from build123d import *

# Parameters (mm, degrees)
SKETCH1_W           = 25.4
SKETCH1_H           = 50.8
SKETCH1_W_2         = 19.05
SKETCH1_H_2         = 44.45
BOSS_EXTRUDE1_DEPTH = 317.5
SKETCH2_R           = 1.905
CUT_EXTRUDE1_DEPTH  = 322.789030267
SKETCH3_R           = 2.1971
SKETCH3_R_2         = 2.8067
CUT_EXTRUDE2_DEPTH  = 322.789030267


with BuildPart() as part:
    # Sketch1 → Boss-Extrude1 (new, symmetric)
    with BuildSketch(Plane.XY):
        Rectangle(SKETCH1_W, SKETCH1_H)
        Rectangle(SKETCH1_W_2, SKETCH1_H_2, mode=Mode.SUBTRACT)
    extrude(amount=BOSS_EXTRUDE1_DEPTH, both=True)

    # Sketch2 → Cut-Extrude1 (cut, through all)
    with BuildSketch(Plane(origin=(0, 25.4, 0), x_dir=(1, 0, 0), z_dir=(0, 1, 0))):
        with Locations(Location((0, -120.1166, 0), (0, 0, 270))):
            Circle(SKETCH2_R)
        with Locations(Location((0, -94.7166, 0), (0, 0, 270))):
            Circle(SKETCH2_R)
        with Locations(Location((0, 235.48594, 0), (0, 0, 270))):
            Circle(SKETCH2_R)
        with Locations(Location((0, 210.08594, 0), (0, 0, 270))):
            Circle(SKETCH2_R)
    extrude(amount=-CUT_EXTRUDE1_DEPTH, mode=Mode.SUBTRACT)

    # Sketch3 → Cut-Extrude2 (cut, through all)
    with BuildSketch(Plane(origin=(0, 25.4, 0), x_dir=(1, 0, 0), z_dir=(0, 1, 0))):
        with Locations((673.1, -279.399917536)):
            Circle(SKETCH3_R)
        with Locations((673.1, -228.599917536)):
            Circle(SKETCH3_R)
        with Locations((673.1, -177.799917536)):
            Circle(SKETCH3_R)
        with Locations(Location((0, -279.399917536, 0), (0, 0, 270))):
            Circle(SKETCH3_R_2)
        with Locations(Location((0, -228.599917536, 0), (0, 0, 270))):
            Circle(SKETCH3_R_2)
        with Locations(Location((0, -177.799917536, 0), (0, 0, 270))):
            Circle(SKETCH3_R_2)
    extrude(amount=-CUT_EXTRUDE2_DEPTH, mode=Mode.SUBTRACT)


solid = part.part
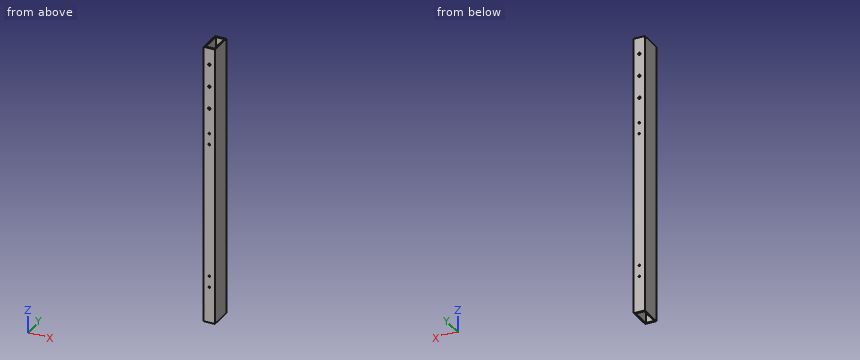
The model under review builds one solid part; all positions refer to its coordinate system, in mm. Coordinates: 2 decimals unless noted, no trailing zeros. Loops run counter-clockwise (first coordinate to the right, second up) from the corner with the lowest first, then second, coordinate; pieces in that order, holes last. Notation, with made-up numbers: M -18,0 L -9,0 A27 cw -9,39 Z; hole C 0,15.5 d6. An arc over 180 degrees is marked long. Put each result on its own line as item: value. Start each with the question number.
Q1. Add section A-A (z = -75). Write out the cut boundary in (x, y) (3 decimals).
Q2. Clearance check with flat-ended pins moving along their axes: pin 1 (6.5 mm diameter, centred on x = 0, z = 279.4, fed in from +Y); pin 2 (4.5 mm diameter, centred on x = 0, z = 228.6, fed in from +Y). State where each tip first meets the part, or that it passes through.
Q3. Wall thickness on line 1 (X direction, y = -5, z = 184) (3 decimals); line 2 (Y direction, x = -2, z = 258.5) (3 decimals): over which ranges is each line inside the solid? List them lowest first.
Q4. Add section B-B (y = 15.5). Write out the cut boundary in (x, z) (3 decimals).
Answers:
1. outline: M -12.7,-25.4 L 12.7,-25.4 L 12.7,25.4 L -12.7,25.4 Z; hole M -9.525,-22.225 L 9.525,-22.225 L 9.525,22.225 L -9.525,22.225 Z
2. pin 1: stops at y = 25.4
2. pin 2: passes through
3. line 1: x = -12.7 to -9.525, 9.525 to 12.7
3. line 2: y = -25.4 to -22.225, 22.225 to 25.4
4. outline: M -12.7,-317.5 L -9.525,-317.5 L -9.525,317.5 L -12.7,317.5 Z; M 9.525,-317.5 L 12.7,-317.5 L 12.7,317.5 L 9.525,317.5 Z
